For this review, take the finished solid that the model builds, in its own axes (mm). Face numbers are marked on the shaded views. Give positions to 0.01 mm unless a question says otherwise; leave off trailing zeros. Write each loop counter-clockwise with the first axis right and the second up, starting at its lowest first coordinate (ties: lowest second). Pieces come first, ordered by that corner, then holes.
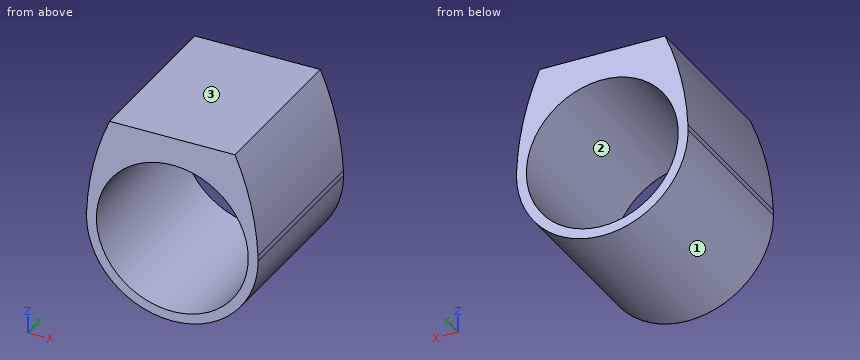
from build123d import *

# Parameters (mm, degrees)
F1_DEPTH = 25


with BuildPart() as f1:
    # F0 (on Front) → F1 (new body)
    with BuildSketch(Plane.XZ):
        with BuildLine():
            ThreePointArc((9.5, 6.4807406984), (10.9886304879, 3.3911649916), (11.5, 0))
            ThreePointArc((11.5, 0), (-3.3911649916, -10.9886304879), (-9.5, 6.4807406984))
            Line((-9.5, 6.4807406984), (-9.5, 8.8741196746))
            ThreePointArc((-9.5, 8.8741196746), (-11.932192643, 5.1597266138), (-12.9726060851, 0.8434994728))
            ThreePointArc((-12.9726060851, 0.8434994728), (-12.9884576775, 0.4218197114), (-13, 0))
            ThreePointArc((-13, 0), (0, -13), (13, 0))
            ThreePointArc((13, 0), (12.9884576775, 0.4218197114), (12.9726060851, 0.8434994728))
            ThreePointArc((12.9726060851, 0.8434994728), (11.932192643, 5.1597266138), (9.5, 8.8741196746))
            Line((9.5, 8.8741196746), (9.5, 6.4807406984))
        make_face()
        with BuildLine():
            ThreePointArc((-9.5, 6.4807406984), (0, 11.5), (9.5, 6.4807406984))
            Line((9.5, 6.4807406984), (9.5, 8.8741196746))
            ThreePointArc((9.5, 8.8741196746), (0, 13), (-9.5, 8.8741196746))
            Line((-9.5, 8.8741196746), (-9.5, 6.4807406984))
        make_face()
        with BuildLine():
            Line((9.5, 15.7431904227), (9.5, 8.8741196746))
            ThreePointArc((9.5, 8.8741196746), (11.932192643, 5.1597266138), (12.9726060851, 0.8434994728))
            ThreePointArc((12.9726060851, 0.8434994728), (11.932253156, 8.45554701), (9.5, 15.7431904227))
        make_face()
        with BuildLine():
            ThreePointArc((-9.5, 8.8741196746), (0, 13), (9.5, 8.8741196746))
            Line((9.5, 8.8741196746), (9.5, 15.7431904227))
            Line((9.5, 15.7431904227), (-9.5, 15.7431904227))
            Line((-9.5, 15.7431904227), (-9.5, 8.8741196746))
        make_face()
        with BuildLine():
            ThreePointArc((-12.9726060851, 0.8434994728), (-11.932192643, 5.1597266138), (-9.5, 8.8741196746))
            Line((-9.5, 8.8741196746), (-9.5, 15.7431904227))
            ThreePointArc((-9.5, 15.7431904227), (-11.932253156, 8.45554701), (-12.9726060851, 0.8434994728))
        make_face()
    extrude(amount=F1_DEPTH)


solid = f1.part
(1) We need section A-A (y = -20.75). Write out the cut boundary in (x, z).
(2) Clearance check with flat-ended pins moving along their axes: pin 1 Ø5 at (y, z) = (-3.5, 3.5) entering from +X; pin 2 Ø3 at (y, z) = (-10, 5.5) entering from -X; pin 3 Ø4 at (x, z) = (6, 6) entering from -Y; pin 4 Ø1.5 at (y, z) = (-2.5, 8) entering from -X. State where each tip first meets the part, or that it passes through.
(3) The part is to be moulded in two halves that separate along X. For the marked faces 1, 2 and 3, say which applies: +X half, -X half, draft (parallel to the pull), parting line (faces both ways), or undercut.
(4) We need section B-B (x = 0). Write out the cut boundary in (y, z).
(5) We need section C-C (z = -4.5). Write out the cut boundary in (x, y).
(6) For L1, parallel to Z at x = 0, y = -18; L2, parallel to Z at x = -1.75, y = -12.25; L3, parallel to X at y = -19.75, z = -2.5, list the stretches that pass through material, from the lowest coordinate up.
The answers:
1. outline: (-13, 0) arc R13 ccw to (13, 0) arc R41.3 ccw to (9.5, 15.74) - (-9.5, 15.74) arc R41.3 ccw to start; hole circle Ø23 at (0, 0)
2. pin 1: stops at x = 12.97
2. pin 2: stops at x = -12.72
2. pin 3: passes through
2. pin 4: stops at x = -12.19
3. face 1: parting line
3. face 2: undercut
3. face 3: draft
4. outline: (-25, -13) - (0, -13) - (0, -11.5) - (-25, -11.5) - close; (-25, 11.5) - (0, 11.5) - (0, 15.74) - (-25, 15.74) - close
5. outline: (-12.2, -25) - (-10.58, -25) - (-10.58, 0) - (-12.2, 0) - close; (10.58, -25) - (12.2, -25) - (12.2, 0) - (10.58, 0) - close
6. L1: z = -13 to -11.5, 11.5 to 15.74
6. L2: z = -12.88 to -11.37, 11.37 to 15.74
6. L3: x = -12.76 to -11.22, 11.22 to 12.76
